from build123d import *

# Parameters (mm, degrees)
BOSS_EXTRUDE1_DEPTH  = 20
SKETCH2_W            = 12.120438769
SKETCH2_H            = 18
CUT_EXTRUDE1_DEPTH   = 26
SKETCH3_R            = 6
CUT_EXTRUDE2_DEPTH   = 5
CUT_EXTRUDE3_REACH   = 66.166
SKETCH4_R            = 3.25
FILLET3_R            = 0.5
FILLET3_OF_MIRROR1_R = 0.5


with BuildPart() as part:
    # Sketch1 → Boss-Extrude1 (new body)
    with BuildSketch(Plane.XY):
        with BuildLine():
            Line((0, 0), (0, 9.76))
            Line((0, 9.76), (14.120438769, 32.578629051))
            ThreePointArc((14.120438769, 32.578629051), (15.211347014, 33.620676168), (16.671503315, 34))
            Line((16.671503315, 34), (52.5, 34))
            Line((52.5, 34), (52.5, 29.35))
            Line((52.5, 29.35), (18, 29.35))
            ThreePointArc((18, 29.35), (15.878679656, 28.471320344), (15, 26.35))
            Line((15, 26.35), (15, 0))
            Line((15, 0), (0, 0))
        make_face()
    boss_extrude1 = extrude(amount=BOSS_EXTRUDE1_DEPTH)

    # Sketch2 → Cut-Extrude1 (cut)
    with BuildSketch(Plane(origin=(0, 34, 0), x_dir=(1, 0, 0), z_dir=(0, 1, 0))):
        with Locations((7.060219385, -10)):
            Rectangle(SKETCH2_W, SKETCH2_H)
    cut_extrude1 = extrude(amount=-CUT_EXTRUDE1_DEPTH, mode=Mode.SUBTRACT)

    # Sketch3 → Cut-Extrude2 (cut)
    with BuildSketch(Plane(origin=(0, 8, 0), x_dir=(1, 0, 0), z_dir=(0, 1, 0))):
        with Locations(Location((7.5, -10, 0), (0, 0, 270))):
            Circle(SKETCH3_R)
    cut_extrude2 = extrude(amount=-CUT_EXTRUDE2_DEPTH, mode=Mode.SUBTRACT)

    # Sketch4 → Cut-Extrude3 (cut, up to next)
    with BuildSketch(Plane(origin=(0, 3, 0), x_dir=(1, 0, 0), z_dir=(0, 1, 0)), mode=Mode.PRIVATE) as cut_extrude3_sk1:
        with Locations(Location((7.5, -10, 0), (0, 0, 270))):
            Circle(SKETCH4_R)
    cut_extrude3_tool1 = extrude(cut_extrude3_sk1.sketch, amount=-CUT_EXTRUDE3_REACH, mode=Mode.PRIVATE) & part.part
    cut_extrude3 = cut_extrude3_tool1.solids().sort_by_distance((7.5, 3, 10))[0]
    add(cut_extrude3, mode=Mode.SUBTRACT)

    # Fillet3
    fillet3_edges = [part.edges().sort_by_distance(p)[0] for p in [
        (15.211347014, 33.620676168, 0),
        (34.585751658, 34, 0),
        (35.25, 29.35, 0),
        (15.878679656, 28.471320344, 0),
        (15, 13.175, 0),
        (7.5, 0, 0),
        (15.878679656, 28.471320344, 20),
        (0, 0, 10),
        (0, 9.76, 10),
        (15, 0, 10),
        (35.25, 29.35, 20),
        (34.585751658, 34, 20),
        (13.120438769, 30.962629051, 10),
        (15.211347014, 33.620676168, 20),
        (7.060219385, 21.169314525, 20),
        (0, 4.88, 20),
        (7.5, 0, 20),
        (15, 13.175, 20),
        (0, 4.88, 0),
        (7.060219385, 21.169314525, 0),
    ]]
    fillet(fillet3_edges, radius=FILLET3_R)

    # Mirror1: Boss-Extrude1, Cut-Extrude1, Cut-Extrude2, Cut-Extrude3 across plane
    add(boss_extrude1.mirror(Plane(origin=(52.5, 34, 20), x_dir=(0, 0, 1), z_dir=(-1, 0, 0))))
    add(cut_extrude1.mirror(Plane(origin=(52.5, 34, 20), x_dir=(0, 0, 1), z_dir=(-1, 0, 0))), mode=Mode.SUBTRACT)
    add(cut_extrude2.mirror(Plane(origin=(52.5, 34, 20), x_dir=(0, 0, 1), z_dir=(-1, 0, 0))), mode=Mode.SUBTRACT)
    add(cut_extrude3.mirror(Plane(origin=(52.5, 34, 20), x_dir=(0, 0, 1), z_dir=(-1, 0, 0))), mode=Mode.SUBTRACT)

    # Fillet3 of Mirror1
    fillet3_of_mirror1_edges = [part.edges().sort_by_distance(p)[0] for p in [
        (89.788652986, 33.620676168, 0),
        (70.414248342, 34, 0),
        (69.75, 29.35, 0),
        (89.121320344, 28.471320344, 0),
        (90, 13.175, 0),
        (97.5, 0, 0),
        (89.121320344, 28.471320344, 20),
        (105, 0, 10),
        (105, 9.76, 10),
        (90, 0, 10),
        (69.75, 29.35, 20),
        (70.414248342, 34, 20),
        (91.879561231, 30.962629051, 10),
        (89.788652986, 33.620676168, 20),
        (97.939780615, 21.169314525, 20),
        (105, 4.88, 20),
        (97.5, 0, 20),
        (90, 13.175, 20),
        (105, 4.88, 0),
        (97.939780615, 21.169314525, 0),
    ]]
    fillet(fillet3_of_mirror1_edges, radius=FILLET3_OF_MIRROR1_R)


solid = part.part
Here's how the part is built. I have some questions about the finished solid (model axes, mm). A direction names the side the tool comes from. Coordinates: 2 decimals unless noted, no trailing zeros. Loops run counter-clockwise (first coordinate to the right, second up) from the corner with the lowest first, then second, coordinate; pieces in that order, holes last.
1. If we mould it in two halves opening along X, with no side actions, what happens to faces 4 (the flat face through (1, 10, 10)), 5 (the cylindrical face through (91.55, 5.54, 9.22)), 6 (the cylindrical face through (89.81, 33.61, 9.87)), 7 (the flat face through (7.065, 21.177, 0.808))? For each: pulls with the +X half, pulls with the -X half, needs draft (parallel to the pull), parting line crosses it, or undercut.
2. I need wall thicknesses on L1, parallel to X at y = 4.35, z = 10; L2, parallel to X at y = 1.2, z = 10; L3, parallel to X at y = 16.5, z = 13.25. Which ranges of each line are inside material? Lowest first, please.
3. For P1, Ø5, axis at y = 18, z = 7, coming from the +X side; P2, Ø3, axis at y = 19, z = 7.5, coming from the -X side; P3, Ø5, axis at x = 7.5, z = 10, coming from the -Y side; P4, Ø2, axis at x = 24, z = 9, coming from the -Y side, each with a flat end and sliding along its axis, tell me the tip position at first contact or that it passes through.
4. Imagine slicing it at B-B, the plane z = 10. Count the separate pieces of the cut face and the enclosed holes in it, and give its area (3 significant figures).
5. For faces 1 (the cylindrical face through (15.19, 33.61, 9.87)), 2 (the flat face through (15, 14, 10)), 3 (the flat face through (104, 10, 10)), which set-ups out of +Z, -Z, +X, -X, +Y, -Y let a thin tool reach every point of the face, with its end or its side?
6. Imagine slicing it at A-A, the plane x = 44. Please give me the cut outline in (y, z).
Taken from the geometry:
1. face 4: undercut
1. face 5: undercut
1. face 6: pulls with the +X half
1. face 7: pulls with the -X half
2. L1: x = 0 to 1.5, 13.5 to 15, 90 to 91.5, 103.5 to 105
2. L2: x = 0 to 4.25, 10.75 to 15, 90 to 94.25, 100.75 to 105
2. L3: x = 13.12 to 15, 90 to 91.88
3. P1: stops at x = 91.88
3. P2: stops at x = 13.12
3. P3: passes through
3. P4: stops at y = 29.35
4. separate pieces: 3
4. enclosed holes: 0
4. area: 530 mm2
5. face 1: +Z, -Z, -X, +Y
5. face 2: +Z, -Z, -Y
5. face 3: +Y
6. outline: (29.35, 0.5) arc R0.5 ccw to (29.85, 0) - (33.5, 0) arc R0.5 ccw to (34, 0.5) - (34, 19.5) arc R0.5 ccw to (33.5, 20) - (29.85, 20) arc R0.5 ccw to (29.35, 19.5) - close
